Verification items for the finished model (mm, model axes). Face numbers are marked on the shaded views. A direction names the side the tool comes from. Round coordinates to 2 decimals unless told otherwise and drop trailing zeros. Write each loop counter-clockwise with the first axis right and the second up, starting at its lowest first coordinate (ties: lowest second). Pieces come first, ordered by that corner, then holes. Notation, with made-up numbers: M 47,-35.75 L 58,-35.75 A20 ccw 58,-27.75 Z; hole C 74,-15 d1. An arc over 180 degrees is marked long. One line per question, with ' | ' between items.
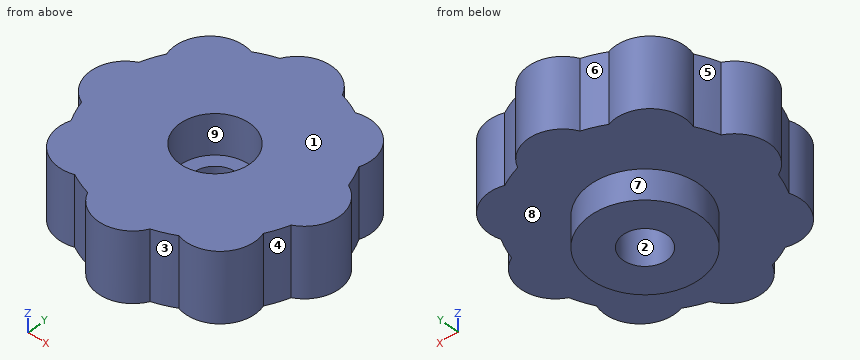
Autodesk Fusion 360 part; units mm, degrees
sketch "Sketch1" plane through (0, 0, 0) normal (0, 0, 1) x (1, 0, 0) in component "Knob"
  circle A0 centre (0, 0) radius 11
  line L0 (0, 0) -> (0, 9) construction
  arc A1 (3.1422, 10.5417) -> (-3.1422, 10.5417) centre (0, 9) ccw
  arc A2 (-5.2322, 9.6759) -> (-9.6759, 5.2322) centre (-6.364, 6.364) ccw
  arc A3 (-10.5417, 3.1422) -> (-10.5417, -3.1422) centre (-9, 0) ccw
  arc A4 (-9.6759, -5.2322) -> (-5.2322, -9.6759) centre (-6.364, -6.364) ccw
  arc A5 (-3.1422, -10.5417) -> (3.1422, -10.5417) centre (0, -9) ccw
  arc A6 (5.2322, -9.6759) -> (9.6759, -5.2322) centre (6.364, -6.364) ccw
  arc A7 (10.5417, -3.1422) -> (10.5417, 3.1422) centre (9, 0) ccw
  arc A8 (9.6759, 5.2322) -> (5.2322, 9.6759) centre (6.364, 6.364) ccw
  circle A9 centre (0, 0) radius 5.5
  circle A10 centre (0, 0) radius 2.2
  circle A11 centre (0, 0) radius 3.5
  dimension "d1" = 22
  dimension "d2" = 7
  dimension "d4" = 360
  dimension "d5" = 11
  dimension "d6" = 4.4
  dimension "d16" = 7
extrude "Extrude1" add sketch "Sketch1" along normal blind 7 contours A0 | A0 A7 | A0 A8 | A0 A6 | A0 A1 | A0 A5 | A0 A2 | A0 A4 | A0 A3 | A9 | A11 in component "Knob"
extrude "Extrude2" add sketch "Sketch1" against normal blind 3 contours A9 | A11 in component "Knob"
extrude "Extrude3" cut sketch "Sketch1" against normal blind 4 from surface at 7 contours A11 in component "Knob"
component "Knob" placed x (1, 0, 0) y (0, 1, 0) z (0, 0, 1) at (0, 0, 0)
1. Section check A-A, the plane y = 0. Record the cut outline in (x, z).
Results:
outline: M -12.5,0 L -5.5,0 L -5.5,-3 L -2.2,-3 L -2.2,3 L -3.5,3 L -3.5,7 L -12.5,7 Z; M 2.2,-3 L 5.5,-3 L 5.5,0 L 12.5,0 L 12.5,7 L 3.5,7 L 3.5,3 L 2.2,3 Z
2. Thickness scan on line 1 (Y direction, x = 0, z = -1.4); line 2 (Y direction, x = 0, z = 5.75); line 3 (Z direction, x = -8.5, y = -8.25). Record the ranges inside material, lowest first.
Results:
line 1: y = -5.5 to -2.2, 2.2 to 5.5 | line 2: y = -12.5 to -3.5, 3.5 to 12.5 | line 3: z = 0 to 7
3. Mould release check, pull along X, two halves, no side actions. Record for the marked faces 6, 7, 8 and 9: pulls with the +X half, pulls with the -X half, needs draft (parallel to the pull), parting line crosses it, or undercut.
Results:
face 6: undercut | face 7: parting line crosses it | face 8: needs draft | face 9: undercut
4. Section check C-C, the plane z = 1.75. Record the cut outline in (x, y).
Results:
outline: M -10.54,-3.14 A11 ccw -9.68,-5.23 A3.5 ccw -5.23,-9.68 A11 ccw -3.14,-10.54 A3.5 ccw 3.14,-10.54 A11 ccw 5.23,-9.68 A3.5 ccw 9.68,-5.23 A11 ccw 10.54,-3.14 A3.5 ccw 10.54,3.14 A11 ccw 9.68,5.23 A3.5 ccw 5.23,9.68 A11 ccw 3.14,10.54 A3.5 ccw -3.14,10.54 A11 ccw -5.23,9.68 A3.5 ccw -9.68,5.23 A11 ccw -10.54,3.14 A3.5 ccw Z; hole C 0,0 d4.4
5. Section check D-D, the plane z = -2. Record the cut outline in (x, y), then the cut area to 3 significant figures.
Results:
outline: C 0,0 d11; hole C 0,0 d4.4 | area: 79.8 mm2
6. Go/stop test with flat-tipped pins: P1, Ø8, axis at x = -9.5, y = 4, coming from the -Z side; P2, Ø2.5, axis at x = 0, y = 0, coming from the +Z side; P3, Ø2, axis at y = -9.5, z = 5, coming from the +X side; P4, Ø1, axis at x = 3, z = 4, coming from the -Y side. Record where each tip stops, or that it passes through.
Results:
P1: stops at z = 0 | P2: passes through | P3: stops at x = 9.14 | P4: stops at y = -11.45
7. Tool access check on the marked faces 1, 2, 3, 4 and 5. Record the directions out of +Z, -Z, +X, -X, +Y, -Y that give a thin tool (end or side, any length) a straight path to the whole face; none if there is none.
Results:
face 1: +Z, +X, -X, +Y, -Y | face 2: +Z, -Z | face 3: +Z, -Z, -Y | face 4: +Z, -Z, +X | face 5: +Z, -Z, -X
